Could you check a few things on this model? Use its own coordinates, in mm. Face numbers are marked on the shaded views. A direction names the side the tool comes from. Give positions to 0.01 mm unless a question says otherwise; leave off trailing zeros. Write each loop counter-clockwise with the first axis right and the second up, starting at its lowest first coordinate (ties: lowest second). Pieces come first, ordered by that corner, then holes. Notation, with made-up numbers: (-12, -12) - (46, -12) arc R26 ccw to (46, 26) - close; hole circle Ø4 at (60.5, 50). An arc over 180 degrees is marked (long way). Write item = value, one per line.
Autodesk Inventor part; units mm, degrees
ref_plane "Work Plane2" through (-1.6732, 2.5, 3.75) normal (0, 0, 1) x (1, 0, 0)
ref_plane "YZ Plane" through (0, 0, 0) normal (1, 0, 0) x (0, 1, 0)
ref_plane "XZ Plane" through (0, 0, 0) normal (0, 1, 0) x (-1, 0, 0)
ref_plane "Work Plane1" through (0, 0, 0) normal (0, 0, 1) x (1, 0, 0)
sketch "Sketch1" plane through (0, 0, 0) normal (0, 0, 1) x (1, 0, 0)
  line L0 (-1.6732, 4.7) -> (-6.6732, 4.7)
  line L1 (8.3268, 7.5) -> (-1.6732, 4.7)
  line L2 (8.3268, 12.5) -> (8.3268, 7.5)
  line L3 (-1.6732, 15.3) -> (8.3268, 12.5)
  line L4 (-6.6732, 15.3) -> (-1.6732, 15.3)
  line L5 (-6.6732, 4.7) -> (-6.6732, 15.3)
  line L6 (-1.7556, 5.3) -> (-6.0732, 5.3)
  line L7 (-6.0732, 5.3) -> (-6.0732, 14.7)
  line L8 (-6.0732, 14.7) -> (-1.7556, 14.7)
  line L9 (-1.7556, 14.7) -> (7.7268, 12.0449)
  line L10 (7.7268, 12.0449) -> (7.7268, 7.9551)
  line L11 (7.7268, 7.9551) -> (-1.7556, 5.3)
  line L12 (7.7268, 12.0449) -> (8.3268, 12.0449)
  line L13 (7.7268, 7.9551) -> (8.3268, 7.9551)
  point P0 (0, 0)
  dimension "d0" = 0.6
ref_plane "Work Plane2" through (-1.6732, 2.5, 3.75) normal (0, 0, 1) x (1, 0, 0)
extrude "Extrusion1" add sketch "Sketch1" along normal blind 3.25 contours L13 L10 L12 L2 | L11 L6 L7 L8 L9 L10
mirror "Mirror2" about plane through (8.3268, 7.9551, 0) normal (1, 0, 0) of "Extrusion1"
properties part number "Bow Tie Key"
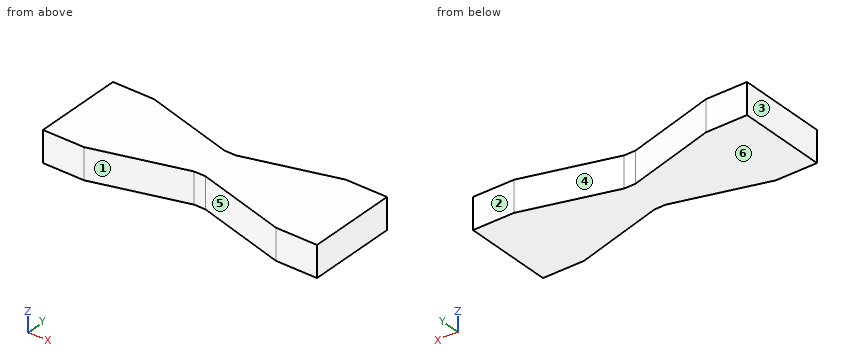
1. Which directions (+Z, -Z, +X, -X, +Y, -Y) give clear straight access to the entire face, cutting with the end or side of a thin tool? Please do the marked faces 4, 5 and 6.
Filled sheet:
face_4 = +Z, -Z, +Y
face_5 = +Z, -Z, -Y
face_6 = -Z, +X, -X, +Y, -Y
2. If we section it at B-B, the plane z = 2.95: Please give me the cut outline in (x, y).
Filled sheet:
outline = (-6.07, 5.3) - (-1.76, 5.3) - (7.73, 7.96) - (8.93, 7.96) - (18.41, 5.3) - (22.73, 5.3) - (22.73, 14.7) - (18.41, 14.7) - (8.93, 12.04) - (7.73, 12.04) - (-1.76, 14.7) - (-6.07, 14.7) - close
3. Thinking about a two-plate mould opening in X: for the marked faces 1, 2 and 3, which applies, pulls with the +X half, pulls with the -X half, needs draft (parallel to the pull), parting line crosses it, or undercut?
Filled sheet:
face_1 = undercut
face_2 = needs draft
face_3 = pulls with the -X half
4. If we section it at A-A, the plane y = 7.5: Please give me the cut outline in (x, z).
Filled sheet:
outline = (-6.07, 0) - (6.1, 0) - (6.1, 3.25) - (-6.07, 3.25) - close; (10.55, 0) - (22.73, 0) - (22.73, 3.25) - (10.55, 3.25) - close
5. If we section it at C-C, the plane x = 11.5: Please give me the cut outline in (y, z), and give its area (3 significant figures).
Filled sheet:
outline = (7.23, 0) - (12.77, 0) - (12.77, 3.25) - (7.23, 3.25) - close
area = 18.0 mm2
6. For pin 1 (1 mm diameter, centred on x = 14, y = 6.5, fed in from +Z); pin 2 (1 mm diameter, centred on x = 8.5, z = 1, fed in from -Y), each with a flat end and sliding along its axis, tell me the tip position at first contact or that it passes through.
Filled sheet:
pin_1 = 3.25
pin_2 = 7.93
7. If we section it at D-D, the plane x = 1.5: Please give me the cut outline in (y, z), and give its area (3 significant figures).
Filled sheet:
outline = (6.21, 0) - (13.79, 0) - (13.79, 3.25) - (6.21, 3.25) - close
area = 24.6 mm2
8. I need wall thicknesses on line 1 (Y direction, x = 8.75, z = 1.45); line 2 (Y direction, x = 18, z = 2). Which ranges of each line are inside material? Lowest first, please.
Filled sheet:
line_1 = 7.96 to 12.04
line_2 = 5.41 to 14.59
